from build123d import *

# Parameters (mm, degrees)
SKETCH_5_R          = 1.8
CUT_EXTRUDE_2_DEPTH = 1.3
FILLET_1_R          = 1
SKETCH_6_R          = 1.693988814
CUT_EXTRUDE_3_DEPTH = 0.5
FILLET_2_R          = 1


with BuildPart() as part:
    # 草图1 → 旋转1 (revolve)
    with BuildSketch(Plane(origin=(0, 0, 0), x_dir=(0, 0, -1), z_dir=(1, 0, 0))):
        Polygon((6.186687636, 3.02056076), (6.186687636, 0), (-6.813312364, 0), (-6.813312364, 3.8), (-3.136442493, 3.8), align=None)
    revolve(axis=Axis((0, 0, -6.352286977), (0, 0, 1)))

    # 草图5 → 切除-拉伸2 (cut)
    with BuildSketch(Plane.XY.offset(6.813312364)):
        Circle(SKETCH_5_R)
    extrude(amount=-CUT_EXTRUDE_2_DEPTH, mode=Mode.SUBTRACT)

    # 圆角1
    fillet_1_edges = [part.edges().sort_by_distance(p)[0] for p in [
        (0, -3.02056076, -6.186687636),
    ]]
    fillet(fillet_1_edges, radius=FILLET_1_R)

    # 草图6 → 切除-拉伸3 (cut)
    with BuildSketch(Plane(origin=(0, 0, -6.186687636), x_dir=(-1, 0, 0), z_dir=(0, 0, -1))):
        with Locations(Location((0, 0, 0), (0, 0, 90))):
            Circle(SKETCH_6_R)
    extrude(amount=-CUT_EXTRUDE_3_DEPTH, mode=Mode.SUBTRACT)

    # 圆角2
    # the kernel refuses this fillet: 1 mm, written as the material it adds along each edge
    with BuildSketch(Plane(origin=(0, 0, -5.686687636), x_dir=(0, 1, 0), z_dir=(-1, 0, 0))) as fillet_2_piece_1:
        with BuildLine():
            CenterArc((0.82796341, 1), FILLET_2_R, 270, 60)
            Line((0.82796341, 0), (0.82796341, -0.02))
            Line((0.82796341, -0.02), (1.693988814, -0.02))
            Line((1.693988814, -0.02), (1.713988814, 0))
            ThreePointArc((1.713988814, 0), (1.713988814, 0.25), (1.711309322, 0.49))
            Line((1.711309322, 0.49), (1.693988814, 0.5))
        make_face()
    revolve(axis=Axis((0, 0, -5.686687636), (0, 0, -1)))


solid = part.part
Model file for the job. Use its own axes, mm. A direction names the side the tool comes from. Give positions to 0.01 mm unless a question says otherwise; leave off trailing zeros. Write each loop counter-clockwise with the first axis right and the second up, starting at its lowest first coordinate (ties: lowest second). Pieces come first, ordered by that corner, then holes. Notation, with made-up numbers: (55, 8.5) -> (101, 8.5) arc R31 ccw to (101, 38.5) -> close; hole circle Ø10 at (-5.5, 69). An arc over 180 degrees is marked (long way). Write item = value, one per line.
(1) Probe line 1 along Y through (x, z) = (0, 6.2); line 2 along Z through (x, y) = (0, 0.75); line 3 along Y through (x, z) = (3, 5.5). List the from-to ranges inside material, lowest first.
Determined:
line_1 = -3.8 to -1.8, 1.8 to 3.8
line_2 = -5.69 to 5.51
line_3 = -2.33 to 2.33
(2) Slice it at B-B, the plane z = -1.25. Give the cut face in (x, y), then the cut area to 3 significant figures.
Determined:
outline = circle Ø6.87 at (0, 0)
area = 37.0 mm2
(3) Flat gauge pins, fed straight in: P1, Ø1.5, axis at y = -3, z = -0.5, coming from the +X side; P2, Ø0.5, axis at x = 0.5, y = 0.5, coming from the -Z side; P3, Ø4, axis at x = 0.5, z = -2.5, coming from the +Y side. Where does each tip first touch, or does it go through?
Determined:
P1 = 2.68
P2 = -5.7
P3 = 3.49
(4) Slice it at A-A, the plane z = 4.75. Give the cut face in (x, y), then the cut area to 3 significant figures.
Determined:
outline = circle Ø7.6 at (0, 0)
area = 45.4 mm2
(5) Mould opens along X. For faces 3 (the face through (-0.167, -3.796, 4.949)), 4 (the face through (1, -2, 6.813)), 5 (the face through (0, 0, -5.687)) say: released by +X, released by -X, zero draft, split by the parting line, or undercut.
Determined:
face_3 = split by the parting line
face_4 = zero draft
face_5 = undercut
(6) Tool access for faces 1 (the face through (2.1, -2.73, -1.13)), 2 (the face through (0, 0, 5.513)): list every direction of +Z, -Z, +X, -X, +Y, -Y with a clear straight run to the whole face (end or side of a thin tool).
Determined:
face_1 = -Z
face_2 = +Z
